For this review, take the finished solid that the model builds, in its own axes (mm). Face numbers are marked on the shaded views. A direction names the side the tool comes from. Round coordinates to 2 decimals unless told otherwise and drop trailing zeros. Order: outer loops, then holes, each group sorted by start corner. A loop starts at its lowest first (then second) coordinate and runs counter-clockwise, first axis right, second up. Notation, with made-up numbers: (30, -9) -> (46, -9) arc R17 cw to (46, 12) -> close; hole circle Ø11 at (6, 51.25). An arc over 180 degrees is marked (long way). Answer in a Markdown table with one row per item.
```python
from build123d import *

# Parameters (mm, degrees)
PAD_DEPTH         = 20
POCKET_DEPTH      = 6.001
POCKET_DEPTH_BACK = -28.001


with BuildPart() as part:
    # AdditivePipe: sweep along a path in Sketch
    with BuildLine(Plane.XY) as additivepipe_path:
        Line((0, 0), (0, 47))
    # Sketch001 → AdditivePipe (sweep)
    with BuildSketch(Plane.XZ):
        Polygon((-20, 6), (-20, -6), (-16, -6), (-9, -6), (9, -6), (16, -6), (20, -6), (20, 6), (16, 6), (16, 3), (9, 3), (9, 6), (-9, 6), (-9, 3), (-16, 3), (-16, 6), align=None)
    sweep(path=additivepipe_path.line)

    # Sketch002 → Pad (new body, symmetric)
    with BuildSketch(Plane.YZ):
        Polygon((47, 3), (47, 14), (34, 28), (22, 28), (22, 14), (29, 14), (29, 3), align=None)
    extrude(amount=PAD_DEPTH, both=True)

    # Sketch003 → Pocket (cut, two sides)
    with BuildSketch(Plane.XY) as pocket_sk:
        with BuildLine():
            ThreePointArc((7, 12.362), (0, 19.362), (-7, 12.362))
            Line((-7, 12.362), (-7, 0))
            Line((-7, 0), (7, 0))
            Line((7, 12.362), (7, 0))
        make_face()
    extrude(amount=-POCKET_DEPTH, mode=Mode.SUBTRACT)
    extrude(pocket_sk.sketch, amount=-POCKET_DEPTH_BACK, mode=Mode.SUBTRACT)


solid = part.part
```
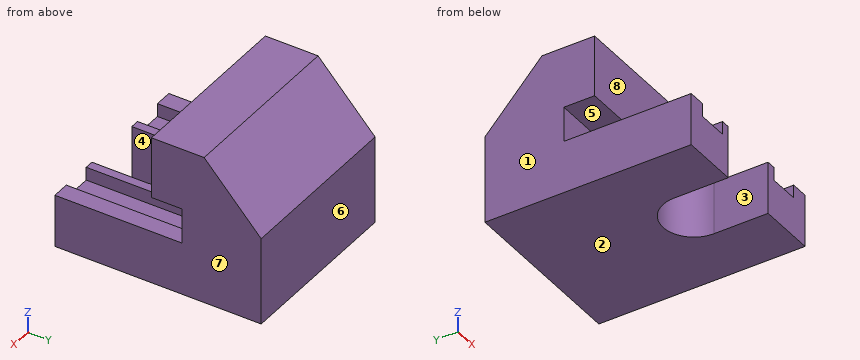
Q1. Clearance check with flat-ended pins moving along their axes: pin 1 Ø4.5 at (x, y) = (-17.5, 20.5) entering from +Z; pin 2 Ø9 at (x, y) = (-4, 12.5) entering from +Z; pin 3 Ø1 at (x, z) = (-9, 17.5) entering from +Y; pin 4 Ø10 at (x, z) = (-16, 19.5) entering from -Y. State where each tip first meets the part, or that it passes through.
Answer key:
| item | result |
|---|---|
| pin 1 | stops at z = 28 |
| pin 2 | stops at z = 6 |
| pin 3 | stops at y = 44.21 |
| pin 4 | stops at y = 22 |
Q2. The part is to be moulded in two halves that separate along X. For the marked faces 1, 2 and 3, say which applies: +X half, -X half, draft (parallel to the pull), parting line (faces both ways), or undercut.
Answer key:
| item | result |
|---|---|
| face 1 | -X half |
| face 2 | draft |
| face 3 | undercut |
Q3. Take a section at C-C, the plane z = 12. Write out the cut boundary in (x, y), then the cut area to 3 significant figures.
Answer key:
| item | result |
|---|---|
| outline | (-20, 29) -> (20, 29) -> (20, 47) -> (-20, 47) -> close |
| area | 720 mm^2 |
Q4. Take a section at D-D, the plane x = 0. Write out the cut boundary in (y, z), then the cut area to 3 significant figures.
Answer key:
| item | result |
|---|---|
| outline | (19.36, -6) -> (47, -6) -> (47, 14) -> (34, 28) -> (22, 28) -> (22, 14) -> (29, 14) -> (29, 6) -> (19.36, 6) -> close |
| area | 735 mm^2 |
Q5. Tool access review of the marked faces 4, 5, 6, 7 and 8: name each direction out of +Z, -Z, +X, -X, +Y, -Y from which nothing blocks a thin tool from reaching the whole face with its end or side.
Answer key:
| item | result |
|---|---|
| face 4 | +Z, -Z, -Y |
| face 5 | +X, -X, -Y |
| face 6 | +Z, -Z, +X, -X, +Y |
| face 7 | +Z, -Z, +X, +Y, -Y |
| face 8 | +Z, +X, -X, -Y |
Q6. Take a section at B-B, the plane y = 18. Write out the cut boundary in (x, z), then the cut area to 3 significant figures.
Answer key:
| item | result |
|---|---|
| outline | (-20, -6) -> (-4.15, -6) -> (-4.15, 6) -> (-9, 6) -> (-9, 3) -> (-16, 3) -> (-16, 6) -> (-20, 6) -> close; (4.15, -6) -> (20, -6) -> (20, 6) -> (16, 6) -> (16, 3) -> (9, 3) -> (9, 6) -> (4.15, 6) -> close |
| area | 338 mm^2 |
Q7. Take a section at A-A, the plane x = -18. Write out the cut boundary in (y, z), then the cut area to 3 significant figures.
Answer key:
| item | result |
|---|---|
| outline | (0, -6) -> (47, -6) -> (47, 14) -> (34, 28) -> (22, 28) -> (22, 14) -> (29, 14) -> (29, 6) -> (0, 6) -> close |
| area | 967 mm^2 |
Q8. To check wall thickness, follow probe 1 along X at (y, z) = (20, 3.5); probe 2 along Z at (x, y) = (14.5, 25); probe 3 along Z at (x, y) = (3, 28). State the ranges of each line that lie inside material, in increasing order.
Answer key:
| item | result |
|---|---|
| probe 1 | x = -20 to -16, -9 to 9, 16 to 20 |
| probe 2 | z = -6 to 3, 14 to 28 |
| probe 3 | z = -6 to 6, 14 to 28 |
